For this review, take the finished solid that the model builds, in its own axes (mm). A direction names the side the tool comes from. Give positions to 0.01 mm unless a question says otherwise; leave off trailing zeros. Loops run counter-clockwise (first coordinate to the right, second up) from the corner with the lowest first, then second, coordinate; pieces in that order, holes last. Notation, with made-up numbers: (-31, -22) -> (8, -22) arc R28 cw to (8, -1) -> close; hole circle Ø11 at (-23, 46). An arc over 180 degrees is marked (long way). Answer as CSV lines item,"result". Start each with the question number.
Item 1: For L1, parallel to Z at x = 4, y = -3.25; L2, parallel to Y at x = -13, z = 18; L3, parallel to X at y = 2.5, z = 31.5, list the stretches that pass through material, from the lowest coordinate up. Write a range as from..to.
Item 2: Add section C-C on z = 57. State the section outline as (x, y) points.
Item 3: Machinability: for faces 5 (the face through (0.105, -13.885, 5.831)), 6 (the face through (-31, 0, 32)), 7 (the face through (7.5, -13, 5)), 8 (the face through (0, 2.7, 33)), which of the approach directions +Z, -Z, +X, -X, +Y, -Y give a long, thin tool a straight path to every point of the face, cutting with its end or side? Answer none if there is none.
Item 4: The part is to be moulded in two halves that separate along X. For faces 1 (the face through (27.971, -9, 4)), 2 (the face through (-7.5, -13, 5)), 3 (the face through (0, 3.5, 32)), 4 (the face through (-5, -18, 1)), say which applies: +X half, -X half, draft (parallel to the pull), parting line (faces both ways), or undercut.
Item 5: Clearance check with flat-ended pins moving along their axes: P1, Ø1.5, axis at x = -16, y = -9.5, coming from the +Z side; P2, Ø1.8, axis at y = -8.5, z = 3, coming from the -X side; P3, Ø10, axis at y = -5.5, z = 21, coming from the -X side; P4, Ø0.6, axis at y = -16.5, z = 1, coming from the +X side. State where each tip first meets the part, or that it passes through.
Item 6: Add section B-B on x = 4. State the section outline as (y, z) points.
Item 7: Add section A-A on y = -17.5. State the section outline as (x, z) points, plus the area to 3 significant figures.
Item 8: Add section D-D on y = 0.5. State the section outline as (x, z) points, plus the area to 3 significant figures.
```python
from build123d import *

# Parameters (mm, degrees)
F0_W     = 60.4
F0_H     = 5.4
F0_W_2   = 10
F0_H_2   = 8
F0_R     = 1.5
F0_W_3   = 1.0285907388
F0_H_3   = 10
F1_DEPTH = 2
F2_DEPTH = 65
F3_R     = 19
F4_DEPTH = 2
F5_DEPTH = 6
F6_W     = 15
F6_H     = 1.6


with BuildPart() as f1:
    # F0 (on Top) → F1 (new body)
    with BuildSketch(Plane.XY):
        Polygon((27.9714092612, -13.5), (27.9714092612, -3.5), (-27.9714092612, -3.5), (-27.9714092612, -13.5), (-5, -13.5), (5, -13.5), align=None)
        Polygon((29, -3.5), (31, -3.5), (31, 3.5), (-31, 3.5), (-31, -3.5), (-29, -3.5), (-27.9714092612, -3.5), (27.9714092612, -3.5), align=None)
        Rectangle(F0_W, F0_H, mode=Mode.SUBTRACT)
        Rectangle(F0_W, F0_H)
        with Locations((0, -17.5)):
            Rectangle(F0_W_2, F0_H_2)
        with Locations((-2.1274185274, -17.5)):
            Circle(F0_R, mode=Mode.SUBTRACT)
        with Locations((-28.4857046306, -8.5)):
            Rectangle(F0_W_3, F0_H_3)
        with Locations((28.4857046306, -8.5)):
            Rectangle(F0_W_3, F0_H_3)
    extrude(amount=F1_DEPTH)

    # F0 (on Top) → F2 (join)
    with BuildSketch(Plane.XY):
        Polygon((29, -3.5), (31, -3.5), (31, 3.5), (-31, 3.5), (-31, -3.5), (-29, -3.5), (-27.9714092612, -3.5), (27.9714092612, -3.5), align=None)
        Rectangle(F0_W, F0_H, mode=Mode.SUBTRACT)
    extrude(amount=F2_DEPTH)

    # F3 (on face) → F4 (cut)
    with BuildSketch(Plane.XZ.offset(3.5)):
        with Locations((4, 30)):
            Circle(F3_R)
    extrude(amount=-F4_DEPTH, mode=Mode.SUBTRACT)

    # F0 (on Top) → F5 (join)
    with BuildSketch(Plane.XY):
        with Locations((28.4857046306, -8.5)):
            Rectangle(F0_W_3, F0_H_3)
        with Locations((-28.4857046306, -8.5)):
            Rectangle(F0_W_3, F0_H_3)
    extrude(amount=F5_DEPTH)

    # F8: sweep along a path in F7
    with BuildLine(Plane.YZ) as f8_path:
        Line((-13.6184291914, 1.5092007816), (-13.6184291914, 4.3010520749))
        ThreePointArc((-13.6184291914, 4.3010520749), (-14.0722220518, 5.726785993), (-15.2666270733, 6.627919618))
    # F6 (on face) → F8 (sweep)
    with BuildSketch(Plane.XY.offset(2)):
        with Locations((0, -12.6052284613)):
            Rectangle(F6_W, F6_H)
    sweep(path=f8_path.line)


solid = f1.part
```
Computed values:
1,L1,"0..11, 49..65"
1,L2,"-3.5..-2.7, 2.7..3.5"
1,L3,"-31..-30.2, 30.2..31"
2,outline,"(-31, -3.5) -> (31, -3.5) -> (31, 3.5) -> (-31, 3.5) -> close; hole (-30.2, -2.7) -> (30.2, -2.7) -> (30.2, 2.7) -> (-30.2, 2.7) -> close"
3,face 5,"-Y"
3,face 6,"+Z, -Z, -X, +Y, -Y"
3,face 7,"+Z, -Y"
3,face 8,"+Z"
4,face 1,"undercut"
4,face 2,"undercut"
4,face 3,"draft"
4,face 4,"-X half"
5,P1,"z = 2"
5,P2,"x = -29"
5,P3,"x = -31"
5,P4,"x = 5"
6,outline,"(-21.5, 0) -> (3.5, 0) -> (3.5, 65) -> (2.7, 65) -> (2.7, 2) -> (-2.7, 2) -> (-2.7, 11) -> (-3.5, 11) -> (-3.5, 2) -> (-11.81, 2) -> (-11.81, 4.3) arc R4.28 ccw to (-14.67, 8.34) -> (-15.2, 6.83) arc R2.68 cw to (-13.41, 4.3) -> (-13.41, 2) -> (-21.5, 2) -> close; (-3.5, 49) -> (-2.7, 49) -> (-2.7, 65) -> (-3.5, 65) -> close"
7,outline,"(-5, 0) -> (-3.63, 0) -> (-3.63, 2) -> (-5, 2) -> close; (-0.63, 0) -> (5, 0) -> (5, 2) -> (-0.63, 2) -> close"
7,area,"14.0 mm²"
8,outline,"(-31, 0) -> (31, 0) -> (31, 65) -> (30.2, 65) -> (30.2, 2) -> (-30.2, 2) -> (-30.2, 65) -> (-31, 65) -> close"
8,area,"225 mm²"
